Design review of the part shown in the three views and the two pictorial views. Dimensions are in mm from the part's minimum x, y and z. A direction names the side the tool comes from. Round coordinates to 2 decimals unless told otherwise and drop trailing zeros. Order: outer loops, then holes, each group sorted by start corner. A loop starts at its lowest first (then second) coordinate and runs counter-clockwise, first axis right, second up.
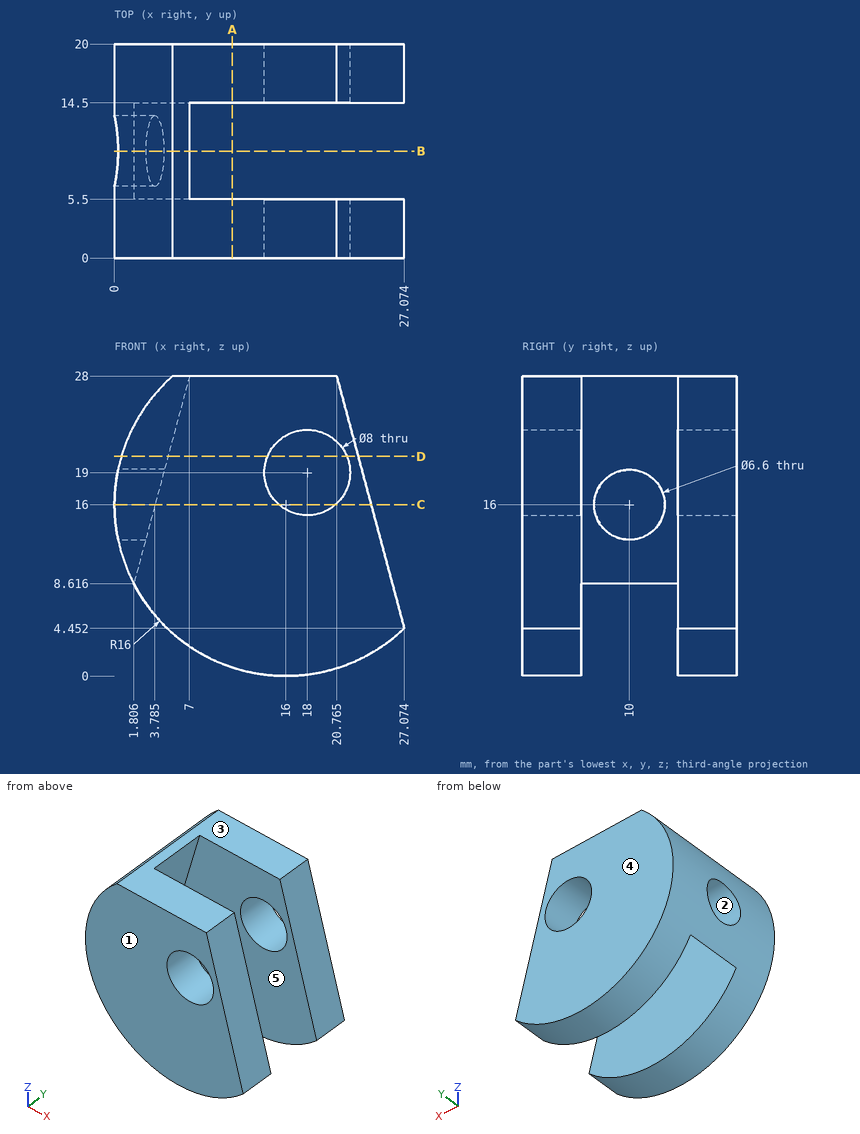
1) To check wall thickness, follow line 1 along Y through (x, z) = (9.5, 13.75); line 2 along X through (y, z) = (18.5, 18.5) (1 decimal); line 3 along Z through (x, y) = (19.5, 1.5). State the ranges of each line that lie inside material, in increasing order.
Results:
line 1: y = 0 to 5.5, 14.5 to 20
line 2: x = 0.2 to 14, 22 to 23.3
line 3: z = 0.39 to 15.29, 22.71 to 28
2) Take a section at C-C on z = 16. Give the boundary of the cut face in (x, y) (1 decimal), plus the area to 3 significant figures.
Results:
outline: (0, 0) - (15.4, 0) - (15.4, 5.5) - (3.8, 5.5) - (3.8, 6.7) - (0, 6.7) - close; (0, 13.3) - (3.8, 13.3) - (3.8, 14.5) - (15.4, 14.5) - (15.4, 20) - (0, 20) - close; (20.6, 0) - (24, 0) - (24, 5.5) - (20.6, 5.5) - close; (20.6, 14.5) - (24, 14.5) - (24, 20) - (20.6, 20) - close
area: 215 mm2
3) Take a section at D-D on z = 20.5. Give the boundary of the cut face in (x, y) (1 decimal).
Results:
outline: (0.6, 0) - (14.3, 0) - (14.3, 5.5) - (5, 5.5) - (5, 14.5) - (14.3, 14.5) - (14.3, 20) - (0.6, 20) - close; (21.7, 0) - (22.8, 0) - (22.8, 5.5) - (21.7, 5.5) - close; (21.7, 14.5) - (22.8, 14.5) - (22.8, 20) - (21.7, 20) - close
4) Take a section at B-B on y = 10. Give the boundary of the cut face in (x, z) (1 decimal).
Results:
outline: (0.3, 12.7) arc R16 ccw to (1.8, 8.6) - (2.9, 12.7) - close; (0.3, 19.3) - (4.7, 19.3) - (7, 28) - (5.4, 28) arc R16 ccw to start
5) Take a section at A-A on x = 11. Give the boundary of the cut face in (y, z), plus the area to 3 significant figures.
Results:
outline: (0, 0.8) - (5.5, 0.8) - (5.5, 28) - (0, 28) - close; (14.5, 0.8) - (20, 0.8) - (20, 28) - (14.5, 28) - close
area: 299 mm2
6) For the marked faces 4 and 5, list the 3-axis set-ups (+Z, -Z, +X, -X, +Y, -Y) from which the entire face can be reached by the end or side of a thin tool; tool diameter is ignored.
Results:
face 4: +Z, -Z, +X, -X, +Y
face 5: -Z, +X
7) The part is to be moulded in two halves that separate along Y. For the marked faces 1, 2 and 3, say which applies: released by +Y, released by -Y, zero draft, split by the parting line, or undercut.
Results:
face 1: released by -Y
face 2: undercut
face 3: zero draft
8) Clearance check with a flat-ended pin moving along its axis: P1, Ø5, axis at x = 5, y = 15, coming from the -Z side (1 decimal). State where the tip first meets the part, or that it passes through.
Results:
P1: stops at z = 2.4
